```python
from build123d import *

# Parameters (mm, degrees)
SKETCH2_R           = 22.5
SKETCH2_R_2         = 2.5
BOSS_EXTRUDE1_DEPTH = 2
CUT_EXTRUDE1_REACH  = 33.883
SKETCH3_R           = 6.05


with BuildPart() as part:
    # Sketch2 → Boss-Extrude1 (new body)
    with BuildSketch(Plane(origin=(0, 0, 0), x_dir=(1, 0, 0), z_dir=(0, 1, 0))):
        with Locations(Location((0, 0, 0), (0, 0, 270))):
            Circle(SKETCH2_R)
        with Locations(Location((-18, 0, 0), (0, 0, 270))):
            Circle(SKETCH2_R_2, mode=Mode.SUBTRACT)
        with Locations(Location((-9, 15.588457268, 0), (0, 0, 270))):
            Circle(SKETCH2_R_2, mode=Mode.SUBTRACT)
        with Locations(Location((9, 15.588457268, 0), (0, 0, 270))):
            Circle(SKETCH2_R_2, mode=Mode.SUBTRACT)
        with Locations(Location((18, 0, 0), (0, 0, 270))):
            Circle(SKETCH2_R_2, mode=Mode.SUBTRACT)
        with Locations(Location((9, -15.588457268, 0), (0, 0, 270))):
            Circle(SKETCH2_R_2, mode=Mode.SUBTRACT)
        with Locations(Location((-9, -15.588457268, 0), (0, 0, 270))):
            Circle(SKETCH2_R_2, mode=Mode.SUBTRACT)
    extrude(amount=BOSS_EXTRUDE1_DEPTH)

    # Sketch3 → Cut-Extrude1 (cut, up to next)
    with BuildSketch(Plane(origin=(0, 2, 0), x_dir=(1, 0, 0), z_dir=(0, 1, 0)), mode=Mode.PRIVATE) as cut_extrude1_sk1:
        with Locations(Location((0, 0, 0), (0, 0, 270))):
            Circle(SKETCH3_R)
    cut_extrude1_tool1 = extrude(cut_extrude1_sk1.sketch, amount=-CUT_EXTRUDE1_REACH, mode=Mode.PRIVATE) & part.part
    add(cut_extrude1_tool1.solids().sort_by_distance((0, 2, 0))[0], mode=Mode.SUBTRACT)


solid = part.part
```
The model under review builds one solid part; all positions refer to its coordinate system, in mm. Give positions to 0.01 mm unless a question says otherwise; leave off trailing zeros. Write each loop counter-clockwise with the first axis right and the second up, starting at its lowest first coordinate (ties: lowest second). Pieces come first, ordered by that corner, then holes.
(1) Consider section C-C, the plane x = -18. Give the boundary of the cut face in (y, z), and give its area (3 significant figures).
(2) Consider section B-B, the plane y = 0.45. Give the boundary of the cut face in (x, z), and give its area (3 significant figures).
(3) For P1, Ø2, axis at x = 11.5, z = -6, coming from the -Y side; P2, Ø4, axis at x = -18, z = 0, coming from the +Y side, all flat-tipped, find the tip position at first contact; note any pin that passes through.
(4) Consider section D-D, the plane z = 14. Give the boundary of the cut face in (x, y), and give its area (3 significant figures).
(5) The part is to be moulded in two halves that separate along Z. For faces 1 (the cylindrical face through (-8.618, 0.986, 20.784)), 2 (the cylindrical face through (-15.52, 0.99, -0.33)), 3 (the flat face through (-5, 0, 5)), say which applies: released by +Z, released by -Z, zero draft, split by the parting line, or undercut.
(6) Consider section A-A, the plane z = 0. Give the boundary of the cut face in (x, y).
(7) To check wall thickness, follow L1, parallel to X at y = 0.7, z = 0; L2, parallel to X at y = 1.3, z = 15; L3, parallel to X at y = 1.6, z = -0.5. State the ranges of each line that lie inside material, in increasing order.
Returned:
1. outline: (0, -13.5) - (2, -13.5) - (2, -2.5) - (0, -2.5) - close; (0, 2.5) - (2, 2.5) - (2, 13.5) - (0, 13.5) - close
1. area: 44.0 mm2
2. outline: circle Ø45 at (0, 0); hole circle Ø5 at (-18, 0); hole circle Ø5 at (-9, -15.59); hole circle Ø5 at (-9, 15.59); hole circle Ø12.1 at (0, 0); hole circle Ø5 at (9, -15.59); hole circle Ø5 at (9, 15.59); hole circle Ø5 at (18, 0)
2. area: 1,360 mm2
3. P1: stops at y = 0
3. P2: passes through
4. outline: (-17.61, 0) - (-10.93, 0) - (-10.93, 2) - (-17.61, 2) - close; (-7.07, 0) - (7.07, 0) - (7.07, 2) - (-7.07, 2) - close; (10.93, 0) - (17.61, 0) - (17.61, 2) - (10.93, 2) - close
4. area: 55.0 mm2
5. face 1: split by the parting line
5. face 2: undercut
5. face 3: zero draft
6. outline: (-22.5, 0) - (-20.5, 0) - (-20.5, 2) - (-22.5, 2) - close; (-15.5, 0) - (-6.05, 0) - (-6.05, 2) - (-15.5, 2) - close; (6.05, 0) - (15.5, 0) - (15.5, 2) - (6.05, 2) - close; (20.5, 0) - (22.5, 0) - (22.5, 2) - (20.5, 2) - close
7. L1: x = -22.5 to -20.5, -15.5 to -6.05, 6.05 to 15.5, 20.5 to 22.5
7. L2: x = -16.77 to -11.43, -6.57 to 6.57, 11.43 to 16.77
7. L3: x = -22.49 to -20.45, -15.55 to -6.03, 6.03 to 15.55, 20.45 to 22.49
